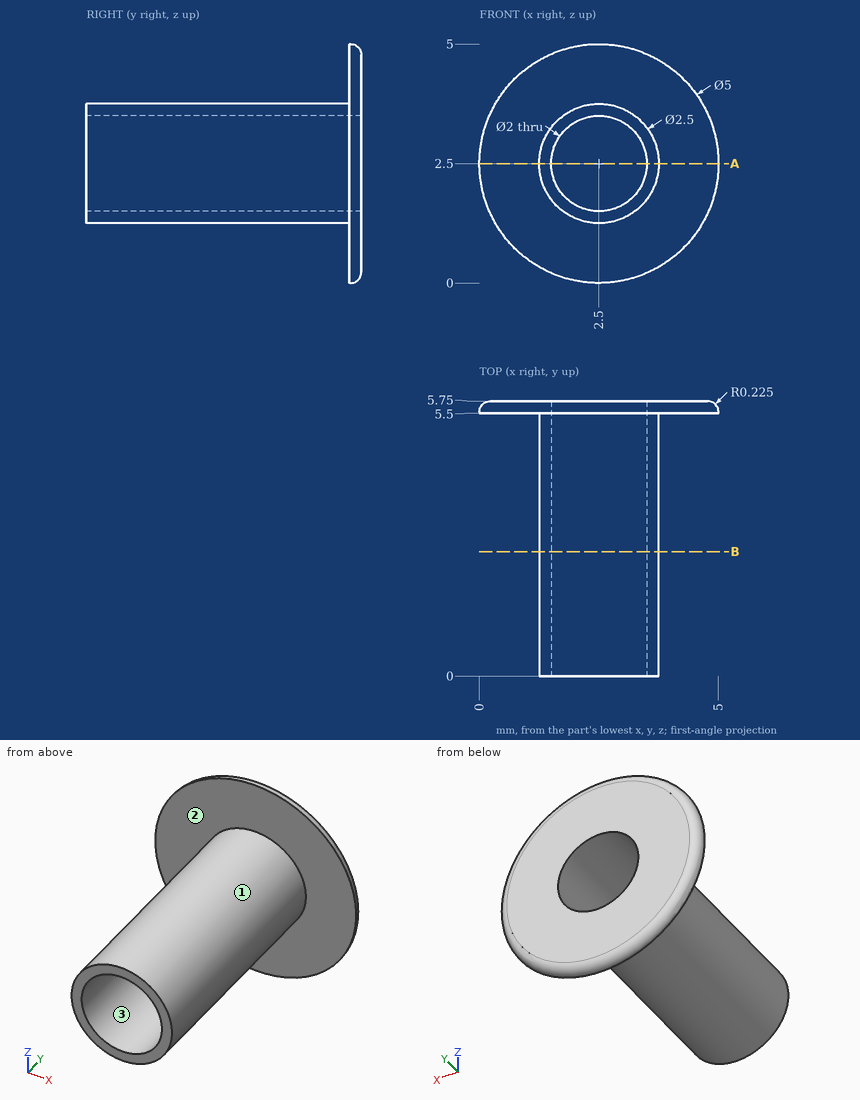
Can you work these out from the drawing? Everything is in mm from the part's minimum corner. Round coordinates to 2 decimals unless told otherwise and drop trailing zeros. Write each loop counter-clockwise with the first axis right and the second up, starting at its lowest first coordinate (ties: lowest second). Pieces come first, ordered by that corner, then holes. Notation, with made-up numbers: M 73.25,-27 L 83.25,-27 A9 ccw 83.25,-23 Z; hole C 53.25,2 d6. An arc over 180 degrees is marked long. Use a Markdown table: item, result.
Item 1: If I drill on line 1 along X through (y, z) = (2.55, 2.5); line 2 along Y through (x, z) = (1.2, 2.6), over which ranges is the centre line in solid material (lowest first)? Write a range as [from, to].
Found:
| item | result |
|---|---|
| line 1 | x = [1.25, 1.5], [3.5, 3.75] |
| line 2 | y = [5.5, 5.75] |
Item 2: We'd pull the mould along Z, two halves only. Please class the marked faces 1, 2 and 3: released by +Z, released by -Z, zero draft, split by the parting line, or undercut.
Found:
| item | result |
|---|---|
| face 1 | split by the parting line |
| face 2 | zero draft |
| face 3 | undercut |
Item 3: For pin 1 Ø2 at (y, z) = (1.5, 4) entering from +X; pin 2 Ø3 at (x, y) = (3, 3) entering from +Z, each with a flat end and sliding along its axis, tell me the tip position at first contact or that it passes through.
Found:
| item | result |
|---|---|
| pin 1 | stops at x = 3.65 |
| pin 2 | stops at z = 3.75 |
Item 4: I want a section at A-A (z = 2.5). List the corners of the cut face in (x, y) for me (3 decimals), and give its area (3 significant figures).
Found:
| item | result |
|---|---|
| outline | M 0,5.5 L 1.25,5.5 L 1.25,0 L 1.5,0 L 1.5,5.75 L 0.225,5.75 A0.225 ccw 0,5.525 Z; M 3.5,0 L 3.75,0 L 3.75,5.5 L 5,5.5 L 5,5.525 A0.225 ccw 4.775,5.75 L 3.5,5.75 Z |
| area | 3.48 mm2 |
Item 5: I want a section at B-B (y = 2.6). List the corners of the cut face in (x, z) for me.
Found:
| item | result |
|---|---|
| outline | C 2.5,2.5 d2.5; hole C 2.5,2.5 d2 |
